from build123d import *

# Parameters (mm, degrees)
SKETCH_1_W          = 70
SKETCH_1_H          = 20
SKETCH_1_R          = 3
EXTRUDE_1_DEPTH     = 3
SKETCH_3_W          = 70
SKETCH_3_H          = 35
EXTRUDE_2_DEPTH     = 3
EXTRUDE_3_DEPTH     = 50
EXTRUDE_4_DEPTH     = 70
SKETCH_6_R          = 5
CUT_EXTRUDE_3_DEPTH = 30
CUT_EXTRUDE_4_DEPTH = 70
SKETCH_8_W          = 15
SKETCH_8_H          = 10
CUT_EXTRUDE_5_DEPTH = 99.615414617


with BuildPart() as part:
    # 草图1 → 凸台-拉伸1 (new body)
    with BuildSketch(Plane.XY):
        Rectangle(SKETCH_1_W, SKETCH_1_H)
        with Locations((-20, 0)):
            Circle(SKETCH_1_R, mode=Mode.SUBTRACT)
        with Locations((20, 0)):
            Circle(SKETCH_1_R, mode=Mode.SUBTRACT)
    extrude(amount=EXTRUDE_1_DEPTH)

    # 草图3 → 凸台-拉伸2 (add)
    with BuildSketch(Plane.XZ.offset(10)):
        with Locations((0, 17.5)):
            Rectangle(SKETCH_3_W, SKETCH_3_H)
    extrude(amount=-EXTRUDE_2_DEPTH)

    # 草图4 → 凸台-拉伸3 (add)
    with BuildSketch(Plane.XZ.offset(10)):
        Polygon((-34, 15), (-31, 35), (-35, 35), (-35, 15), (-35, 0), (-34, 0), align=None)
        Polygon((35, 0), (34, 0), (34, 15), (31, 35), (35, 35), (35, 15), align=None)
    extrude(amount=EXTRUDE_3_DEPTH)

    # 草图5 → 凸台-拉伸4 (add)
    with BuildSketch(Plane.ZY.offset(35)):
        Polygon((3, 10), (3, -7), (35, -7), align=None)
    extrude(amount=-EXTRUDE_4_DEPTH)

    # 草图6 → 切除-拉伸3 (cut)
    with BuildSketch(Plane(origin=(0, 0, 3), x_dir=(-1, 0, 0), z_dir=(0, 0, -1))):
        with Locations((-20, 0)):
            Circle(SKETCH_6_R)
        with Locations((20, 0)):
            Circle(SKETCH_6_R)
    extrude(amount=-CUT_EXTRUDE_3_DEPTH, mode=Mode.SUBTRACT)

    # 草图7 → 切除-拉伸4 (cut)
    with BuildSketch(Plane.ZY.offset(35)):
        Polygon((0, 10), (35, -7), (3, 10), align=None)
    extrude(amount=-CUT_EXTRUDE_4_DEPTH, mode=Mode.SUBTRACT)

    # 草图8 → 切除-拉伸5 (cut, through all)
    with BuildSketch(Plane.ZY.offset(35)):
        with Locations((7.5, -55)):
            Rectangle(SKETCH_8_W, SKETCH_8_H)
    extrude(amount=-CUT_EXTRUDE_5_DEPTH, mode=Mode.SUBTRACT)


solid = part.part
Build history of the part. All positions in model axes, mm. A direction names the side the tool comes from. Give positions to 0.01 mm unless a question says otherwise; leave off trailing zeros. Order: outer loops, then holes, each group sorted by start corner. A loop starts at its lowest first (then second) coordinate and runs counter-clockwise, first axis right, second up. Notation, with made-up numbers: M 28,20 L 71,20 A24 ccw 71,43 Z; hole C -14.5,-31 d2. An arc over 180 degrees is marked long. Use one line per item in the form item = value.
Q1. Pin check, flat tips, straight feed: P1, Ø11.5, axis at x = 20, y = 0, coming from the +Z side; P2, Ø12, axis at x = -23.5, y = -42, coming from the -Z side; P3, Ø3, axis at x = 18.5, z = 9, coming from the +Y side; P4, Ø0.5, axis at x = -34.5, y = -54.5, coming from the -Z side. Stop position of each tip, or through.
Conclusion:
P1 = 32.43
P2 = through
P3 = 6.36
P4 = 15
Q2. Slice it at A-A, the plane y = -55. Write the cut outline in (x, z), and give its area (3 significant figures).
Conclusion:
outline = M -35,15 L -34,15 L -31,35 L -35,35 Z; M 31,35 L 34,15 L 35,15 L 35,35 Z
area = 100 mm2
Q3. Slice it at D-D, the plane z = 22.5. Write the cut outline in (x, y) (3 decimals), and give its area (3 significant figures).
Conclusion:
outline = M -35,-60 L -32.875,-60 L -32.875,-10 L 32.875,-10 L 32.875,-60 L 35,-60 L 35,-0.929 L 24.913,-0.929 A5 cw 15.087,-0.929 L -15.087,-0.929 A5 cw -24.913,-0.929 L -35,-0.929 Z
area = 787 mm2
Q4. Wall check: probe 1 along X at (y, z) = (0, 12.5); probe 2 along X at (y, z) = (-4.5, 13); probe 3 along Y at (x, z) = (20, 1.55). Give the ranges that are in metal, low to high.
Conclusion:
probe_1 = -35 to -25, -15 to 15, 25 to 35
probe_2 = -35 to -22.18, -17.82 to 17.82, 22.18 to 35
probe_3 = -10 to -3, 3 to 9.25
Q5. Slice it at C-C, the plane x = -20. Write the cut outline in (y, z), and give its area (3 significant figures).
Conclusion:
outline = M -10,0 L -3,0 L -3,3 L -5,3 L -5,30.88 L -7,35 L -10,35 Z; M 3,0 L 10,0 L 5,10.29 L 5,3 L 3,3 Z
area = 209 mm2
Q6. Which spindle directions (+Z, -Z, +X, -X, +Y, -Y) get a long thin tool onto all of the face, cutting with end or side? Do faces 4 (the flat face through (34, -30, 7)), 5 (the cylindrical face through (-18.92, -4.88, 13.74)), 6 (the flat face through (-0.49, 1.619, 17.255)). Say none if no direction does.
Conclusion:
face_4 = -Z, -Y
face_5 = +Z
face_6 = +Z, +X, -X, +Y
Q7. Pull direction Y, two halves, no side cores. Call faces 1 (the flat face through (20.1, -3.3, 3)), 2 (the flat face through (-33, -60, 27)), 3 (the flat face through (-32.52, -34.65, 24.86)): released by +Y, released by -Y, zero draft, split by the parting line, or undercut.
Conclusion:
face_1 = undercut
face_2 = released by -Y
face_3 = zero draft
Q8. Slice it at B-B, the plane y = 0. Write the cut outline in (x, z).
Conclusion:
outline = M -35,0 L -23,0 L -23,3 L -25,3 L -25,20.59 L -35,20.59 Z; M -17,0 L 17,0 L 17,3 L 15,3 L 15,20.59 L -15,20.59 L -15,3 L -17,3 Z; M 23,0 L 35,0 L 35,20.59 L 25,20.59 L 25,3 L 23,3 Z
